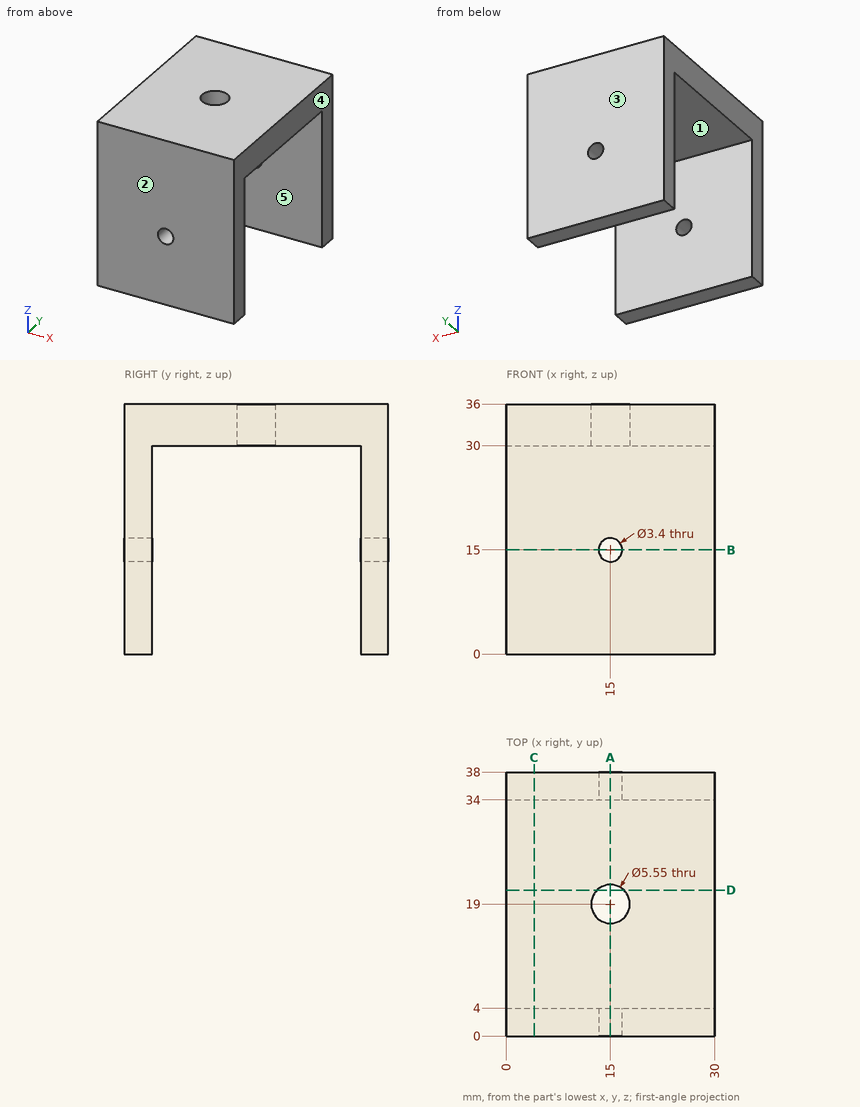
Part print with two shaded views. Sizes in mm from the minimum x, y, z corner. A direction names the side the tool comes from. Coordinates: 2 decimals unless noted, no trailing zeros. Write each loop counter-clockwise with the first axis right and the second up, starting at its lowest first coordinate (ties: lowest second). Pieces come first, ordered by that corner, then holes.
1. Band-saw the part on C-C, the plane x = 4. Give the cut face in (y, z), and give its area (3 significant figures).
Answer block:
outline: (0, 0) - (4, 0) - (4, 30) - (34, 30) - (34, 0) - (38, 0) - (38, 36) - (0, 36) - close
area: 468 mm2
2. Band-saw the part on D-D, the plane y = 21. Give the cut face in (x, z), and give its area (3 significant figures).
Answer block:
outline: (0, 30) - (13.08, 30) - (13.08, 36) - (0, 36) - close; (16.92, 30) - (30, 30) - (30, 36) - (16.92, 36) - close
area: 157 mm2
3. Drop flat-ended pins along their axis: pin 1 (1 mm diameter, centred on x = 5, y = 15.5, fed in from -Z); pin 2 (5 mm diameter, centred on x = 15, y = 19, fed in from -Z) (3 decimals). Give the stop position or say it passes through.
Answer block:
pin 1: stops at z = 30
pin 2: passes through
4. Pull direction Y, two halves, no side cores. Call the marked faces 1, 2 and 3: released by +Y, released by -Y, zero draft, split by the parting line, or undercut.
Answer block:
face 1: undercut
face 2: released by -Y
face 3: released by +Y
5. Drill centre lines: probe 1 along Y at (x, z) = (23.5, 11.5); probe 2 along Y at (x, z) = (15, 33.9) (3 decimals); probe 3 along Z at (x, y) = (28.5, 18.5). Where is each one in solid material? Low to high.
Answer block:
probe 1: y = 0 to 4, 34 to 38
probe 2: y = 0 to 16.225, 21.775 to 38
probe 3: z = 30 to 36
6. 3-axis set-ups, long thin cutter, end or side, ignore diameter. For the marked faces 4 and 5: which of +Z, -Z, +X, -X, +Y, -Y reach the whole face in a straight line?
Answer block:
face 4: +Z, -Z, +X, +Y, -Y
face 5: -Z, +X, -X
7. Band-saw the part on A-A, the plane x = 15. Give the cut face in (y, z) (3 decimals).
Answer block:
outline: (0, 0) - (4, 0) - (4, 13.3) - (0, 13.3) - close; (0, 16.7) - (4, 16.7) - (4, 30) - (16.225, 30) - (16.225, 36) - (0, 36) - close; (21.775, 30) - (34, 30) - (34, 16.7) - (38, 16.7) - (38, 36) - (21.775, 36) - close; (34, 0) - (38, 0) - (38, 13.3) - (34, 13.3) - close
8. Band-saw the part on B-B, the plane z = 15. Give the cut face in (x, y), and give its area (3 significant figures).
Answer block:
outline: (0, 0) - (13.3, 0) - (13.3, 4) - (0, 4) - close; (0, 34) - (13.3, 34) - (13.3, 38) - (0, 38) - close; (16.7, 0) - (30, 0) - (30, 4) - (16.7, 4) - close; (16.7, 34) - (30, 34) - (30, 38) - (16.7, 38) - close
area: 213 mm2
